from build123d import *

# Parameters (mm, degrees)
F0_W     = 120
F0_H     = 28
F1_DEPTH = 5
F2_W     = 28.5
F2_H     = 28
F3_DEPTH = 6.56
F5_R     = 1.3
F6_DEPTH = 11.56
F7_DEPTH = 5
F8_R     = 3
F8_R_2   = 1.3
F9_DEPTH = 1.5


with BuildPart() as f1:
    # F0 (on Front) → F1 (new body)
    with BuildSketch(Plane.XZ):
        with Locations((60, 14)):
            Rectangle(F0_W, F0_H)
    extrude(amount=F1_DEPTH)

    # F2 (on face) → F3 (join)
    with BuildSketch(Plane.XZ.offset(5)):
        with Locations((105.75, 14)):
            Rectangle(F2_W, F2_H)
    extrude(amount=F3_DEPTH)

    # F5 (on face) → F6 (cut, through all)
    with BuildSketch(Plane.XZ.offset(11.56)):
        with Locations((100, 14)):
            Circle(F5_R)
    extrude(amount=-F6_DEPTH, mode=Mode.SUBTRACT)

    # F4 (on face) → F7 (cut, through all)
    with BuildSketch(Plane.XZ.offset(5)):
        with BuildLine():
            ThreePointArc((4.68391, 14.125), (4.680978, 14.062531), (4.68, 14))
            Line((4.68, 14), (4.695687, 14))
            ThreePointArc((4.695687, 14), (4.688817, 14.062408), (4.68391, 14.125))
        make_face()
        with BuildLine():
            ThreePointArc((40.68, 14.25), (40.683925, 14.124754), (40.695687, 14))
            Line((40.695687, 14), (59.664313, 14))
            ThreePointArc((59.664313, 14), (59.676075, 14.124754), (59.68, 14.25))
            ThreePointArc((59.68, 14.25), (59.094214, 15.664214), (57.68, 16.25))
            Line((57.68, 16.25), (42.68, 16.25))
            ThreePointArc((42.68, 16.25), (41.265786, 15.664214), (40.68, 14.25))
        make_face()
        with BuildLine():
            Line((59.664313, 14), (40.695687, 14))
            ThreePointArc((40.695687, 14), (41.357124, 12.75), (42.68, 12.25))
            Line((42.68, 12.25), (57.68, 12.25))
            ThreePointArc((57.68, 12.25), (59.002876, 12.75), (59.664313, 14))
        make_face()
        with BuildLine():
            Line((4.68, 14.25), (4.68, 14))
            ThreePointArc((4.68, 14), (4.680978, 14.062531), (4.68391, 14.125))
            ThreePointArc((4.68391, 14.125), (4.680978, 14.187469), (4.68, 14.25))
        make_face()
        with BuildLine():
            ThreePointArc((4.68391, 14.125), (4.688817, 14.062408), (4.695687, 14))
            Line((4.695687, 14), (23.664313, 14))
            ThreePointArc((23.664313, 14), (23.671183, 14.062408), (23.67609, 14.125))
            ThreePointArc((23.67609, 14.125), (23.049306, 15.457738), (21.68, 16))
            Line((21.68, 16), (6.68, 16))
            ThreePointArc((6.68, 16), (5.310694, 15.457738), (4.68391, 14.125))
        make_face()
        with BuildLine():
            Line((23.664313, 14), (4.695687, 14))
            ThreePointArc((4.695687, 14), (5.357124, 12.75), (6.68, 12.25))
            Line((6.68, 12.25), (21.68, 12.25))
            ThreePointArc((21.68, 12.25), (23.002876, 12.75), (23.664313, 14))
        make_face()
        with BuildLine():
            ThreePointArc((23.67609, 14.125), (23.671183, 14.062408), (23.664313, 14))
            Line((23.664313, 14), (23.68, 14))
            ThreePointArc((23.68, 14), (23.679022, 14.062531), (23.67609, 14.125))
        make_face()
        with BuildLine():
            ThreePointArc((23.67609, 14.125), (23.679022, 14.062531), (23.68, 14))
            Line((23.68, 14), (23.68, 14.25))
            ThreePointArc((23.68, 14.25), (23.679022, 14.187469), (23.67609, 14.125))
        make_face()
    extrude(amount=-F7_DEPTH, mode=Mode.SUBTRACT)

    # F8 (on face) → F9 (cut)
    with BuildSketch(Plane(origin=(0, 0, 0), x_dir=(-1, 0, 0), z_dir=(0, 1, 0))):
        with Locations((-100, 14)):
            Circle(F8_R)
        with Locations((-100, 14)):
            Circle(F8_R_2, mode=Mode.SUBTRACT)
    extrude(amount=-F9_DEPTH, mode=Mode.SUBTRACT)


solid = f1.part
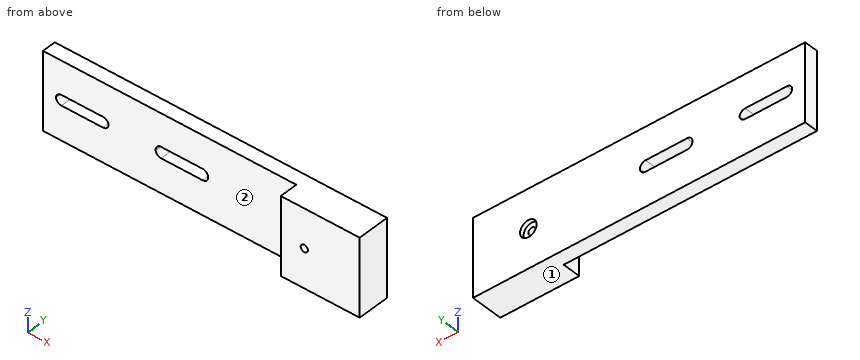
For this review, take the finished solid that the model builds, in its own axes (mm). Face numbers are marked on the shaded views. A direction names the side the tool comes from. Give positions to 0.01 mm unless a question says otherwise; leave off trailing zeros. Loops run counter-clockwise (first coordinate to the right, second up) from the corner with the lowest first, then second, coordinate; pieces in that order, holes last. Notation, with made-up numbers: (11, 75) - (25, 75) arc R13 cw to (25, 94) - close; hole circle Ø6 at (14, 20.5). An arc over 180 degrees is marked (long way). Write each question's results on one line, items separated by ' | '.
(1) Take a section at B-B (y = -6.5). Give the boundary of the cut face in (x, z).
Conclusion:
outline: (91.5, 0) - (120, 0) - (120, 28) - (91.5, 28) - close; hole circle Ø2.6 at (100, 14)
(2) Take a section at D-D (x = 33.5). Give the boundary of the cut face in (y, z), then the cut area to 3 significant figures.
Conclusion:
outline: (-5, 0) - (0, 0) - (0, 28) - (-5, 28) - close | area: 140 mm^2
(3) For the marked faces 1 and 2, list the 3-axis set-ups (+Z, -Z, +X, -X, +Y, -Y) from which the entire face can be reached by the end or side of a thin tool; tool diameter is ignored.
Conclusion:
face 1: -Z, +X, -X, +Y, -Y | face 2: +Z, -Z, -X, -Y
(4) For pin 1 Ø1 at (y, z) = (-1.5, 7) entering from -X; pin 2 Ø3 at (x, z) = (26.5, 23.5) entering from -Y; pin 3 Ø4 at (y, z) = (-8.5, 20) entering from -X; pin 4 Ø5.5 at (x, z) = (100, 14) entering from +Y, all flat-tipped, find the tip position at first contact; note any pin that passes through.
Conclusion:
pin 1: x = 0 | pin 2: y = -5 | pin 3: x = 91.5 | pin 4: y = -1.5
(5) Take a section at A-A (x = 100). Give the boundary of the cut face in (y, z), then the cut area to 3 significant figures.
Conclusion:
outline: (-11.56, 0) - (0, 0) - (0, 11) - (-1.5, 11) - (-1.5, 12.7) - (-11.56, 12.7) - close; (-11.56, 15.3) - (-1.5, 15.3) - (-1.5, 17) - (0, 17) - (0, 28) - (-11.56, 28) - close | area: 289 mm^2
(6) Take a section at C-C (z = 21.75). Give the boundary of the cut face in (x, y).
Conclusion:
outline: (0, -5) - (91.5, -5) - (91.5, -11.56) - (120, -11.56) - (120, 0) - (0, 0) - close
(7) For line 1 along Z through (x, y) = (100, -0.45); line 2 along Z through (x, y) = (99, -5); line 3 along X through (y, z) = (-3, 14.5), list the stretches that pass through material, from the lowest coordinate up.
Conclusion:
line 1: 0 to 11, 17 to 28 | line 2: 0 to 13.17, 14.83 to 28 | line 3: 0 to 4.74, 23.62 to 40.7, 59.66 to 98.8, 101.2 to 120
